Check sheet for the drawn part. Datum: minimum x, y, z corner. Units: mm. A direction names the side the tool comes from. Coordinates: 2 decimals unless noted, no trailing zeros. Loops run counter-clockwise (first coordinate to the right, second up) from the corner with the lowest first, then second, coordinate; pieces in that order, holes last. Notation, with made-up numbers: (44, -22) - (77, -22) arc R26 cw to (77, -7) - close; hole circle Ø1 at (41.5, 35.25). An arc over 180 degrees is marked (long way). Write item = value, one per line. Start each with the question number.
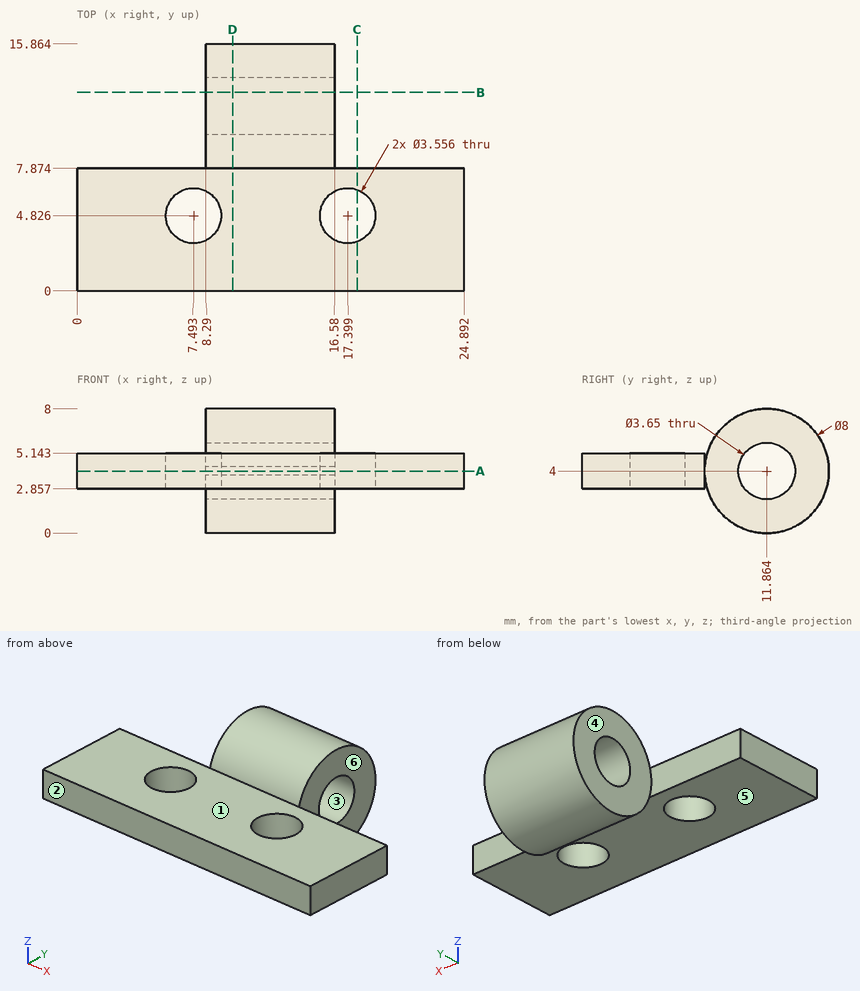
(1) Depth check by flat-ended pin: pin 1 (4 mm diameter, centred on x = 7.493, y = 4.826, fed in from -Z); pin 2 (8 mm diameter, centred on x = 13, y = 5.5, fed in from +Z); pin 3 (4 mm diameter, centred on y = 10.5, z = 4, fed in from +X); pin 4 (2 mm diameter, centred on x = 17.399, y = 4.826, fed in from +Z). Enter the tip coordinate at first touch or a pass-through.
(2) Draft check along Z on the marked faces 1, 2 and 3. Enter one of: pulls with the +Z half, pulls with the -Z half, needs draft (parallel to the pull), parting line crosses it, or undercut.
(3) Scan lines: line 1 (Z direction, x = 17.75, y = 1.5); line 2 (Y direction, x = 10.75, z = 4); line 3 (Y direction, x = 24, z = 3.5). Record each from-to range of solid material in increasing order.
(4) Sectioned sample at A-A on z = 4. Enter the section's corners in (x, y) (3 decimals), plus the area to 3 significant figures.
(5) Sectioned sample at D-D on x = 10. Enter the section's corners in (y, z) (3 decimals), plus the area to 3 significant figures.
(6) Sectioned sample at C-C on x = 18. Enter the section's corners in (y, z), plus the area to 3 significant figures.
(7) Tool access check on the marked faces 4, 5 and 6. Record the directions out of +Z, -Z, +X, -X, +Y, -Y that give a thin tool (end or side, any length) a straight path to the whole face; none if there is none.
(8) Sectioned sample at B-B on y = 12.75. Enter the section's corners in (x, z), plus the area to 3 significant figures.
Working result:
q1.pin_1 = 2.86
q1.pin_2 = 7.23
q1.pin_3 = 16.58
q1.pin_4 = through
q2.face_1 = pulls with the +Z half
q2.face_2 = needs draft
q2.face_3 = undercut
q3.line_1 = 2.86 to 5.14
q3.line_2 = 0 to 10.04, 13.69 to 15.86
q3.line_3 = 0 to 7.87
q4.outline = (0, 0) - (24.892, 0) - (24.892, 7.874) - (16.58, 7.874) - (16.58, 10.039) - (8.29, 10.039) - (8.29, 7.874) - (0, 7.874) - close; (8.29, 13.689) - (16.58, 13.689) - (16.58, 15.864) - (8.29, 15.864) - close; hole circle Ø3.556 at (7.493, 4.826); hole circle Ø3.556 at (17.399, 4.826)
q4.area = 212 mm2
q5.outline = (0, 2.857) - (7.874, 2.857) - (7.874, 3.717) arc R4 ccw (long way) to (7.874, 4.283) - (7.874, 5.143) - (0, 5.143) - close; hole circle Ø3.65 at (11.864, 4)
q5.area = 57.8 mm2
q6.outline = (0, 2.86) - (3.15, 2.86) - (3.15, 5.14) - (0, 5.14) - close; (6.5, 2.86) - (7.87, 2.86) - (7.87, 5.14) - (6.5, 5.14) - close
q6.area = 10.3 mm2
q7.face_4 = +Z, -Z, -X, +Y
q7.face_5 = -Z, +X, -X, -Y
q7.face_6 = +Z, -Z, +X, +Y
q8.outline = (8.29, 0.1) - (16.58, 0.1) - (16.58, 2.4) - (8.29, 2.4) - close; (8.29, 5.6) - (16.58, 5.6) - (16.58, 7.9) - (8.29, 7.9) - close
q8.area = 38.2 mm2
